Model file for the job. Use its own axes, mm. Round coordinates to 2 decimals unless told otherwise and drop trailing zeros. Loops run counter-clockwise (first coordinate to the right, second up) from the corner with the lowest first, then second, coordinate; pieces in that order, holes last. Notation, with made-up numbers: M -39.5,-7.5 L -28.5,-7.5 A26 ccw -28.5,18.5 Z; hole C -8,71.25 d9. An arc over 180 degrees is marked long. Use a Markdown table: item, result. Add a question column.
Item 1: Pin check, flat tips, straight feed: P1, Ø3.5, axis at x = -42, z = -50, coming from the +Y side; P2, Ø4.5, axis at x = 54, z = -50, coming from the +Y side (3 decimals). Stop position of each tip, or through.
Item 2: Saw through at C-C on x = 0. Write the cut outline in (y, z) (3 decimals), then the cut area to 3 significant figures.
Item 3: Saw through at A-A on x = -42. Write the cut outline in (y, z) (3 decimals).
Item 4: Wall check: L1, parallel to X at y = 2.4, z = 50; L2, parallel to Z at x = -42, y = 1.3; L3, parallel to Z at x = 0, y = 1.3. Give the ranges that are in metal, low to high. Write a range as from..to.
Item 5: Saw through at B-B on z = -50. Write the cut outline in (x, y) (3 decimals).
Item 6: Saw through at D-D on y = 2.55. Give the number of separate pieces and of enclosed holes in the cut face, then the cut area to 3 significant figures.
Autodesk Inventor part; units mm, degrees
ref_plane "YZ Plane" through (0, 0, 0) normal (1, 0, 0) x (0, 1, 0)
ref_plane "XZ Plane" through (0, 0, 0) normal (0, 1, 0) x (-1, 0, 0)
ref_plane "XY Plane" through (0, 0, 0) normal (0, 0, 1) x (1, 0, 0)
sketch "Sketch1" plane through (0, 0, 0) normal (0, 1, 0) x (-1, 0, 0)
  line L0 (-60, 75) -> (60, 75)
  line L1 (60, 75) -> (60, -75)
  line L2 (60, -75) -> (-60, -75)
  line L3 (-60, -75) -> (-60, 75)
  line L4 (-60, 75) -> (60, -75) construction
  line L5 (60, 75) -> (-60, -75) construction
  point P0 (0, 0)
  dimension "d0" = 120
  dimension "d1" = 150
extrude "Extrusion1" add sketch "Sketch1" along normal blind 3.175
sketch "Sketch2" plane through (0, 3.175, 0) normal (0, 1, 0) x (1, 0, 0)
  circle A0 centre (-48, -56) radius 2.5 construction
  circle A1 centre (-54, -62) radius 2
  circle A2 centre (-42, -62) radius 2
  circle A3 centre (-42, -50) radius 2
  circle A4 centre (-54, -50) radius 2
  line L0 (-60, 75) -> (-60, -75) construction
  line L1 (-60, 0) -> (60, 0) construction
  line L2 (60, -75) -> (60, 75) construction
  line L3 (-60, -75) -> (60, -75) construction
  line L4 (0, -75) -> (0, 72.2302) construction
  circle A5 centre (-54, 62) radius 2
  circle A6 centre (-42, 62) radius 2
  circle A7 centre (-42, 50) radius 2
  circle A8 centre (-54, 50) radius 2
  circle A9 centre (54, -62) radius 2
  circle A10 centre (42, -62) radius 2
  circle A11 centre (42, -50) radius 2
  circle A12 centre (54, -50) radius 2
  circle A13 centre (42, 50) radius 2
  circle A14 centre (54, 50) radius 2
  circle A15 centre (42, 62) radius 2
  circle A16 centre (54, 62) radius 2
  circle A17 centre (0, 0) radius 7 construction
  circle A18 centre (0, 20) radius 7
  circle A19 centre (0, -20) radius 7
  point P0 (0, 0)
  dimension "d4" = 5
  dimension "d5" = 56
  dimension "d6" = 48
  dimension "d7" = 4
  dimension "d8" = 6
  dimension "d9" = 6
  dimension "d12" = 360
  dimension "d14" = 14
  dimension "d17" = 14
  dimension "d20" = 20
  dimension "d21" = 14
  dimension "d22" = 20
extrude "Extrusion2" cut sketch "Sketch2" against normal through all
properties part number "TurretMotorCase_TopPlate"
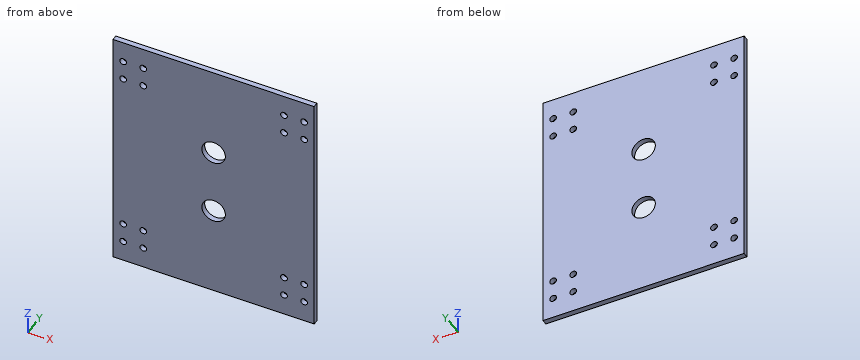
Entries:
| question | item | result |
|---|---|---|
| 1 | P1 | through |
| 1 | P2 | y = 3.175 |
| 2 | outline | M 0,-75 L 3.175,-75 L 3.175,-27 L 0,-27 Z; M 0,-13 L 3.175,-13 L 3.175,13 L 0,13 Z; M 0,27 L 3.175,27 L 3.175,75 L 0,75 Z |
| 2 | area | 387 mm2 |
| 3 | outline | M 0,-75 L 3.175,-75 L 3.175,-64 L 0,-64 Z; M 0,-60 L 3.175,-60 L 3.175,-52 L 0,-52 Z; M 0,-48 L 3.175,-48 L 3.175,48 L 0,48 Z; M 0,52 L 3.175,52 L 3.175,60 L 0,60 Z; M 0,64 L 3.175,64 L 3.175,75 L 0,75 Z |
| 4 | L1 | -60..-56, -52..-44, -40..40, 44..52, 56..60 |
| 4 | L2 | -75..-64, -60..-52, -48..48, 52..60, 64..75 |
| 4 | L3 | -75..-27, -13..13, 27..75 |
| 5 | outline | M -60,0 L -56,0 L -56,3.175 L -60,3.175 Z; M -52,0 L -44,0 L -44,3.175 L -52,3.175 Z; M -40,0 L 40,0 L 40,3.175 L -40,3.175 Z; M 44,0 L 52,0 L 52,3.175 L 44,3.175 Z; M 56,0 L 60,0 L 60,3.175 L 56,3.175 Z |
| 6 | separate pieces | 1 |
| 6 | enclosed holes | 18 |
| 6 | area | 17,500 mm2 |
